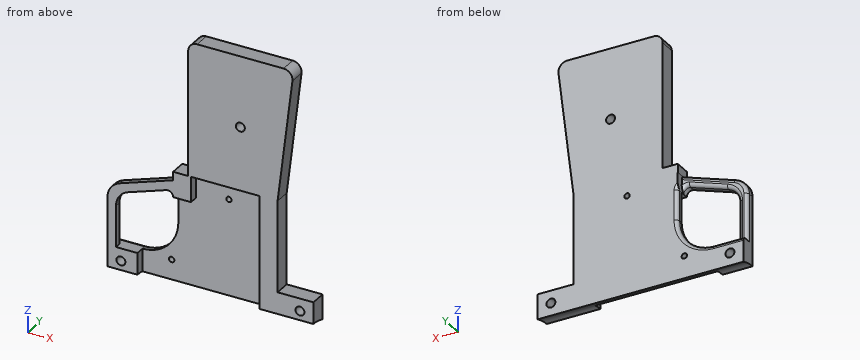
from build123d import *

# Parameters (mm, degrees)
SALIENTE_EXTRUIR1_DEPTH      = 4
REDONDEO1_R                  = 20
REDONDEO2_R                  = 10
REDONDEO3_R                  = 3
CROQUIS2_R                   = 1.5
CORTAR_EXTRUIR1_DEPTH        = 4
SALIENTE_EXTRUIR2_DEPTH      = 5
SALIENTE_EXTRUIR2_DEPTH_BACK = 4
CROQUIS4_W                   = 16.725121099
CROQUIS4_H                   = 14
SALIENTE_EXTRUIR3_DEPTH      = 5
SALIENTE_EXTRUIR4_DEPTH      = 5
CORTAR_EXTRUIR2_START        = -4
CORTAR_EXTRUIR2_DEPTH        = 4
SALIENTE_EXTRUIR5_DEPTH      = 9
REDONDEO4_R                  = 5
CORTAR_EXTRUIR3_DEPTH        = 115
CROQUIS10_R                  = 2.5
CORTAR_EXTRUIR4_DEPTH        = 10
REDONDEO5_R                  = 2


with BuildPart() as part:
    # Croquis1 → Saliente-Extruir1 (new body)
    with BuildSketch(Plane(origin=(0, 0, 0), x_dir=(1, 0, 0), z_dir=(0, 1, 0))):
        Polygon((36.657146199, 0.467319271), (95, 0.467319271), (95, 65.467319271), (0, 65.467319271), (0, 17.557539605), (36.657146199, 5.214366653), align=None)
        Polygon((4.725121099, 51.467319271), (36.725121099, 51.467319271), (36.725121099, 10.467319271), (4.725121099, 21.242340663), align=None, mode=Mode.SUBTRACT)
    extrude(amount=SALIENTE_EXTRUIR1_DEPTH)

    # Redondeo1
    redondeo1_edges = [part.edges().sort_by_distance(p)[0] for p in [
        (36.725121099, 2, -51.467319271),
    ]]
    fillet(redondeo1_edges, radius=REDONDEO1_R)

    # Redondeo2
    redondeo2_edges = [part.edges().sort_by_distance(p)[0] for p in [
        (0, 2, -17.557539605),
        (4.725121099, 2, -21.242340663),
    ]]
    fillet(redondeo2_edges, radius=REDONDEO2_R)

    # Redondeo3
    redondeo3_edges = [part.edges().sort_by_distance(p)[0] for p in [
        (36.725121099, 2, -10.467319271),
    ]]
    fillet(redondeo3_edges, radius=REDONDEO3_R)

    # Croquis2 → Cortar-Extruir1 (cut)
    with BuildSketch(Plane(origin=(0, 4, 0), x_dir=(1, 0, 0), z_dir=(0, 1, 0))):
        with Locations(Location((33, 53, 0), (0, 0, 270))):
            Circle(CROQUIS2_R)
        with Locations(Location((65, 10.467319271, 0), (0, 0, 270))):
            Circle(CROQUIS2_R)
    extrude(amount=-CORTAR_EXTRUIR1_DEPTH, mode=Mode.SUBTRACT)

    # Croquis3 → Saliente-Extruir2 (add, two sides: drawn at the far end of the back side and taken through both)
    with BuildSketch(Plane.XZ.offset(-SALIENTE_EXTRUIR2_DEPTH_BACK)):
        Polygon((95, -0.467319271), (95, -51.467319271), (115, -51.467319271), (115, -65.467319271), (85, -65.467319271), (85, -0.467319271), align=None)
    extrude(amount=SALIENTE_EXTRUIR2_DEPTH + SALIENTE_EXTRUIR2_DEPTH_BACK)

    # Croquis4 → Saliente-Extruir3 (add)
    with BuildSketch(Plane.XZ):
        with Locations((8.36256055, -58.467319271)):
            Rectangle(CROQUIS4_W, CROQUIS4_H)
    extrude(amount=SALIENTE_EXTRUIR3_DEPTH)

    # Croquis5 → Saliente-Extruir4 (add)
    with BuildSketch(Plane.XZ):
        with BuildLine():
            Line((6.808855565, -15.264865719), (36.657146199, -5.214366653))
            Line((36.657146199, -5.214366653), (36.657146199, -0.467319271))
            Line((36.657146199, -0.467319271), (46.657146199, -0.467319271))
            Line((46.657146199, -0.467319271), (46.657146199, -14.642982178))
            Line((46.657146199, -14.642982178), (36.725121099, -14.642982178))
            ThreePointArc((36.725121099, -14.642982178), (35.475545335, -12.206588327), (32.767777769, -11.799833616))
            Line((32.767777769, -11.799833616), (11.533976664, -18.949666776))
            ThreePointArc((11.533976664, -18.949666776), (6.603808263, -22.592081199), (4.725121099, -28.426828651))
            Line((4.725121099, -28.426828651), (4.725121099, -51.467319271))
            Line((4.725121099, -51.467319271), (0, -51.467319271))
            Line((0, -51.467319271), (0, -24.742027593))
            ThreePointArc((0, -24.742027593), (1.878687164, -18.907280142), (6.808855565, -15.264865719))
        make_face()
    extrude(amount=SALIENTE_EXTRUIR4_DEPTH)

    # Cortar-Extruir2: read off the stored shape, not the designer's step
    # Cortar-Extruir2 outline → Cortar-Extruir2 (cut)
    with BuildSketch(Plane(origin=(0, 4, 0), x_dir=(1, 0, 0), z_dir=(0, 1, 0)).offset(CORTAR_EXTRUIR2_START)):
        with BuildLine():
            Line((4.725121099, 51.467319271), (0, 51.467319271))
            Line((0, 51.467319271), (0, 24.742027593))
            ThreePointArc((0, 24.742027593), (1.878687164, 18.907280142), (6.808855565, 15.264865719))
            Line((6.808855565, 15.264865719), (36.657146199, 5.214366653))
            Line((36.657146199, 5.214366653), (36.72480926, 14.599727874))
            ThreePointArc((36.72480926, 14.599727874), (35.457935304, 12.194032416), (32.767777769, 11.799833616))
            Line((32.767777769, 11.799833616), (11.533976664, 18.949666776))
            ThreePointArc((11.533976664, 18.949666776), (6.603808263, 22.592081199), (4.725121099, 28.426828651))
            Line((4.725121099, 28.426828651), (4.725121099, 51.467319271))
        make_face()
    extrude(amount=CORTAR_EXTRUIR2_DEPTH, mode=Mode.SUBTRACT)

    # Croquis8 → Saliente-Extruir5 (add)
    with BuildSketch(Plane(origin=(0, 4, 0), x_dir=(1, 0, 0), z_dir=(0, 1, 0))):
        Polygon((45.08, -74.552680729), (103.96, -74.552680729), (95, 0.467319271), (45.08, 0.467319271), align=None)
    extrude(amount=-SALIENTE_EXTRUIR5_DEPTH)

    # Redondeo4
    redondeo4_edges = [part.edges().sort_by_distance(p)[0] for p in [
        (45.08, -0.5, 74.552680729),
        (103.96, -0.5, 74.552680729),
    ]]
    fillet(redondeo4_edges, radius=REDONDEO4_R)

    # Croquis9 → Cortar-Extruir3 (cut)
    with BuildSketch(Plane(origin=(115, 0, 0), x_dir=(0, 0, -1), z_dir=(1, 0, 0))):
        with BuildLine():
            Line((65.467319271, 4), (65.467319271, -5))
            Line((65.467319271, -5), (63.588909898, -5))
            ThreePointArc((63.588909898, -5), (64.063517857, -0.403033017), (65.467319271, 4))
        make_face()
    extrude(amount=-CORTAR_EXTRUIR3_DEPTH, mode=Mode.SUBTRACT)

    # Croquis10 → Cortar-Extruir4 (cut)
    with BuildSketch(Plane(origin=(0, 4, 0), x_dir=(1, 0, 0), z_dir=(0, 1, 0))):
        with Locations(Location((7.5, 58.467319271, 0), (0, 0, 270))):
            Circle(CROQUIS10_R)
        with Locations(Location((107.5, 58.467319271, 0), (0, 0, 270))):
            Circle(CROQUIS10_R)
        with Locations(Location((74.21, -35, 0), (0, 0, 270))):
            Circle(CROQUIS10_R)
    extrude(amount=-CORTAR_EXTRUIR4_DEPTH, mode=Mode.SUBTRACT)

    # Redondeo5
    # the kernel refuses this fillet: 2 mm, written as the material it takes off along each edge
    with BuildSketch(Plane(origin=(6.808855565, 0, -15.264865719), x_dir=(-3.003248393768829e-11, -1.0, 8.919142254990751e-11), z_dir=(0.9477161874303269, 0, 0.31911444355046886))) as redondeo5_piece_1_section:
        with BuildLine():
            CenterArc((REDONDEO5_R, REDONDEO5_R), REDONDEO5_R, 180.000000005, 90)
            Line((-REDONDEO5_R * 9.41119543218e-11, REDONDEO5_R), (0, 0))
            Line((0, 0), (REDONDEO5_R, 0))
        make_face()
    redondeo5_piece_1 = extrude(amount=36.494967618, mode=Mode.PRIVATE)
    redondeo5_piece_1 = split(redondeo5_piece_1, bisect_by=Plane(origin=(36.728049447, 0, -15.049165525), z_dir=(-0.9999740131061556, 0, -0.007209237988178882)), keep=Keep.TOP, mode=Mode.PRIVATE)
    add(redondeo5_piece_1, mode=Mode.SUBTRACT)
    with BuildSketch(Plane(origin=(9.999999999, 0, -24.742027593), x_dir=(-1.0, 0, 6.147260478780798e-12), z_dir=(-6.147260478780798e-12, 0, -1.0))) as redondeo5_piece_2:
        with BuildLine():
            CenterArc((9.999999999 - REDONDEO5_R, -REDONDEO5_R), REDONDEO5_R, 0, 90)
            Line((9.999999999 + REDONDEO5_R * 5.85513859619e-11, -REDONDEO5_R), (9.999999999, 0))
            Line((9.999999999, 0), (9.999999999 - REDONDEO5_R, 0))
        make_face()
    revolve(axis=Axis((9.999999999, 0, -24.742027593), (0, 1, 0)), revolution_arc=71.390621361, mode=Mode.SUBTRACT)
    with BuildSketch(Plane(origin=(0, 0, -51.467319271), x_dir=(0, -1, 0), z_dir=(0, 0, 1))) as redondeo5_piece_3:
        with BuildLine():
            CenterArc((REDONDEO5_R, REDONDEO5_R), REDONDEO5_R, 180, 90)
            Line((0, REDONDEO5_R), (0, 0))
            Line((0, 0), (REDONDEO5_R, 0))
        make_face()
    extrude(amount=26.725291678, mode=Mode.SUBTRACT)
    with BuildSketch(Plane(origin=(4.725121099, 0, -28.426828651), x_dir=(-1, 0, 0), z_dir=(0, 0, -1))) as redondeo5_piece_4:
        with BuildLine():
            CenterArc((REDONDEO5_R, -REDONDEO5_R), REDONDEO5_R, 90, 90)
            Line((-REDONDEO5_R * 1.16604059741e-10, -REDONDEO5_R), (0, 0))
            Line((0, 0), (REDONDEO5_R, 0))
        make_face()
    extrude(amount=23.04049062, mode=Mode.SUBTRACT)
    with BuildSketch(Plane(origin=(14.725121098, 0, -28.42682865), x_dir=(-0.3191144434609787, 0, 0.94771618746046), z_dir=(0.94771618746046, 0, 0.3191144434609787))) as redondeo5_piece_5:
        with BuildLine():
            CenterArc((9.999999999 + REDONDEO5_R, REDONDEO5_R), REDONDEO5_R, 180, 90)
            Line((9.999999999 - REDONDEO5_R * 2.13431938789e-10, REDONDEO5_R), (9.999999999, 0))
            Line((9.999999999, 0), (9.999999999 + REDONDEO5_R, 0))
        make_face()
    revolve(axis=Axis((14.725121098, 0, -28.42682865), (0, -1, 0)), revolution_arc=71.390621366, mode=Mode.SUBTRACT)
    with BuildSketch(Plane(origin=(32.767777769, 0, -11.799833616), x_dir=(-0.3191144435113306, 0, 0.9477161874435055), z_dir=(-0.9477161874435056, 0, -0.3191144435113306))) as redondeo5_piece_6:
        with BuildLine():
            CenterArc((REDONDEO5_R, -REDONDEO5_R), REDONDEO5_R, 90, 90)
            Line((0, -REDONDEO5_R), (0, 0))
            Line((0, 0), (REDONDEO5_R, 0))
        make_face()
    extrude(amount=22.405232058, mode=Mode.SUBTRACT)
    with BuildSketch(Plane(origin=(33.725121101, 0, -14.642982175), x_dir=(-0.08231883672192833, 0, -0.996606045095427), z_dir=(-0.996606045095427, 0, 0.08231883672192833))) as redondeo5_piece_7_section:
        with BuildLine():
            CenterArc((2.999999998 + REDONDEO5_R, REDONDEO5_R), REDONDEO5_R, 180, 90)
            Line((2.999999998 + REDONDEO5_R, 0), (2.999999998, 0))
            Line((2.999999998, 0), (2.999999998 - REDONDEO5_R * 4.36447322727e-10, REDONDEO5_R))
        make_face()
    redondeo5_piece_7 = revolve(axis=Axis((33.725121101, 0, -14.642982175), (0, -1, 0)), revolution_arc=203.331243748, mode=Mode.PRIVATE)
    redondeo5_piece_7 = split(redondeo5_piece_7, bisect_by=Plane(origin=(36.724965179, 0, -14.621355023), z_dir=(-0.9999740131061556, 0, -0.007209237988178882)), keep=Keep.TOP, mode=Mode.PRIVATE)
    add(redondeo5_piece_7, mode=Mode.SUBTRACT)
    with BuildSketch(Plane(origin=(4.725121099, 4, -51.467319271), x_dir=(0, 0, -1), z_dir=(1, 0, 0))) as redondeo5_piece_8:
        with BuildLine():
            CenterArc((REDONDEO5_R, -REDONDEO5_R), REDONDEO5_R, 90, 90)
            Line((0, -REDONDEO5_R), (0, 0))
            Line((0, 0), (REDONDEO5_R, 0))
        make_face()
    extrude(amount=12, mode=Mode.SUBTRACT)
    with BuildSketch(Plane(origin=(16.725121099, 4, -31.467319271), x_dir=(0, 0, -1), z_dir=(-1, 0, 0))) as redondeo5_piece_9:
        with BuildLine():
            CenterArc((20 + REDONDEO5_R, REDONDEO5_R), REDONDEO5_R, 180, 90)
            Line((20, REDONDEO5_R), (20, 0))
            Line((20, 0), (20 + REDONDEO5_R, 0))
        make_face()
    revolve(axis=Axis((16.725121099, 4, -31.467319271), (0, -1, 0)), revolution_arc=90, mode=Mode.SUBTRACT)
    with BuildSketch(Plane(origin=(36.725121099, 4, -31.467319271), x_dir=(1, 0, 0), z_dir=(0, 0, 1))) as redondeo5_piece_10:
        with BuildLine():
            CenterArc((REDONDEO5_R, -REDONDEO5_R), REDONDEO5_R, 90, 90)
            Line((0, -REDONDEO5_R), (0, 0))
            Line((0, 0), (REDONDEO5_R, 0))
        make_face()
    extrude(amount=16.824337093, mode=Mode.SUBTRACT)
    with BuildSketch(Plane(origin=(33.725121099, 4, -14.642982178), x_dir=(-0.11006554678443577, 0, 0.9939243308275753), z_dir=(-0.9939243308275753, 0, -0.11006554678443577))) as redondeo5_piece_11:
        with BuildLine():
            CenterArc((3 + REDONDEO5_R, -REDONDEO5_R), REDONDEO5_R, 90, 90)
            Line((3, -REDONDEO5_R), (3, 0))
            Line((3, 0), (3 + REDONDEO5_R, 0))
        make_face()
    revolve(axis=Axis((33.725121099, 4, -14.642982178), (0, 1, 0)), revolution_arc=96.319094067, mode=Mode.SUBTRACT)
    with BuildSketch(Plane(origin=(4.725121099, 4, -51.467319271), x_dir=(0, 0, -1), z_dir=(-1, 0, 0))) as redondeo5_piece_12:
        with BuildLine():
            CenterArc((REDONDEO5_R, REDONDEO5_R), REDONDEO5_R, 180, 90)
            Line((-REDONDEO5_R * 1.79170456249e-10, REDONDEO5_R), (0, 0))
            Line((0, 0), (REDONDEO5_R, 0))
        make_face()
    extrude(amount=9.725121099, mode=Mode.SUBTRACT)


solid = part.part
Read the model definition and answer for the solid it produces. Units are mm, in the model's axes. Coordinates: 2 decimals unless noted, no trailing zeros. Order: outer loops, then holes, each group sorted by start corner. A loop starts at its lowest first (then second) coordinate and runs counter-clockwise, first axis right, second up. Notation, with made-up numbers: (-40, 19.5) -> (14, 19.5) arc R21 ccw to (14, 27.5) -> close; hole circle Ø8 at (17, 26.5). An arc over 180 degrees is marked (long way). Answer as a JSON object with one key per item and string values.
1) A cutting plane is placed at C-C, the plane x = 107.5. Determine the outline of the cut face in (y, z).
Model answer:
{"outline": "(-5, -63.59) arc R22.5 cw to (4, -65.47) -> (4, -60.97) -> (-5, -60.97) -> close; (-5, -55.97) -> (4, -55.97) -> (4, -51.47) -> (-5, -51.47) -> close"}
2) A cutting plane is placed at A-A, the plane x = 74.21. Determine the outline of the cut face in (y, z).
Model answer:
{"outline": "(-5, -0.47) -> (0, -0.47) -> (0, -64.15) arc R22.5 cw to (4, -65.47) -> (4, 32.5) -> (-5, 32.5) -> close; (-5, 37.5) -> (4, 37.5) -> (4, 74.55) -> (-5, 74.55) -> close"}
3) Consider line 1 along X through (y, z) = (-0.25, -2); line 2 along X through (y, z) = (-3.5, -45); line 3 along Z through (x, y) = (37, -4.5). Determine where each line is inside the solid, lowest interval first. Write a range as from..to.
Model answer:
{"line 1": "x = 36.66..46.66, 85..95", "line 2": "x = 0..4.73, 85..95", "line 3": "z = -14.64..-0.47"}
4) A cutting plane is placed at D-D, the plane x = 58.5. Determine the outline of the cut face in (y, z).
Model answer:
{"outline": "(-5, -0.47) -> (0, -0.47) -> (0, -64.15) arc R22.5 cw to (4, -65.47) -> (4, 74.55) -> (-5, 74.55) -> close"}
5) A cutting plane is placed at B-B, the plane z = 35. Determine the outline of the cut face in (x, y).
Model answer:
{"outline": "(45.08, -5) -> (71.71, -5) -> (71.71, 4) -> (45.08, 4) -> close; (76.71, -5) -> (99.24, -5) -> (99.24, 4) -> (76.71, 4) -> close"}
6) Each of these flat-tipped pins is pushed along its axis until it touches: pin 1 (4.5 mm diameter, centred on y = -2, z = -22.5, fed in from +X); pin 2 (2 mm diameter, centred on y = 1.5, z = -26.5, fed in from -X); pin 3 (3.5 mm diameter, centred on x = 8, y = -1, fed in from +Z). Where does it stop, or does it pass through?
Model answer:
{"pin 1": "stops at x = 95", "pin 2": "stops at x = 36.73", "pin 3": "stops at z = -14.35"}
